For this review, use the dimensioned drawing (mm, ordinates from the lowest corner) and the shaded views. A direction names the side the tool comes from. Coordinates: 2 decimals unless noted, no trailing zeros. Loops run counter-clockwise (first coordinate to the right, second up) from the corner with the lowest first, then second, coordinate; pieces in that order, holes last. Notation, with made-up numbers: M 81,-23 L 125,-23 A27 cw 125,5 Z; hole C 69.5,72.25 d7. An arc over 180 degrees is marked long. Use CSV: the item, a comma, the result in double quotes. Start each with the question number.
1. Clearance check with flat-ended pins moving along their axes: P1, Ø10, axis at x = 8.5, y = 6.5, coming from the +Z side; P2, Ø14, axis at x = 3, y = 55, coming from the +Z side; P3, Ø8, axis at x = 32.5, z = 27.5, coming from the -Y side. State where each tip first meets the part, or that it passes through.
2. Add section A-A, the plane y = 31. Write out the cut boundary in (x, z).
3. Draft analysis for pull direction Y (two halves, no side actions). For the marked faces 4, 5 and 6, state which applies: +Y half, -Y half, draft (parallel to the pull), parting line (faces both ways), or undercut.
4. Tool access review of the marked faces 1, 2 and 3: name each direction out of +Z, -Z, +X, -X, +Y, -Y from which nothing blocks a thin tool from reaching the whole face with its end or side.
5. For L1, parallel to Y at x = 26, z = 4.5; L2, parallel to X at y = 25, z = 8; L3, parallel to Y at x = 17, z = 28, list the stretches that pass through material, from the lowest coordinate up.
6. Add section C-C, the plane x = 19.5. Write out the cut boundary in (y, z) (1 decimal).
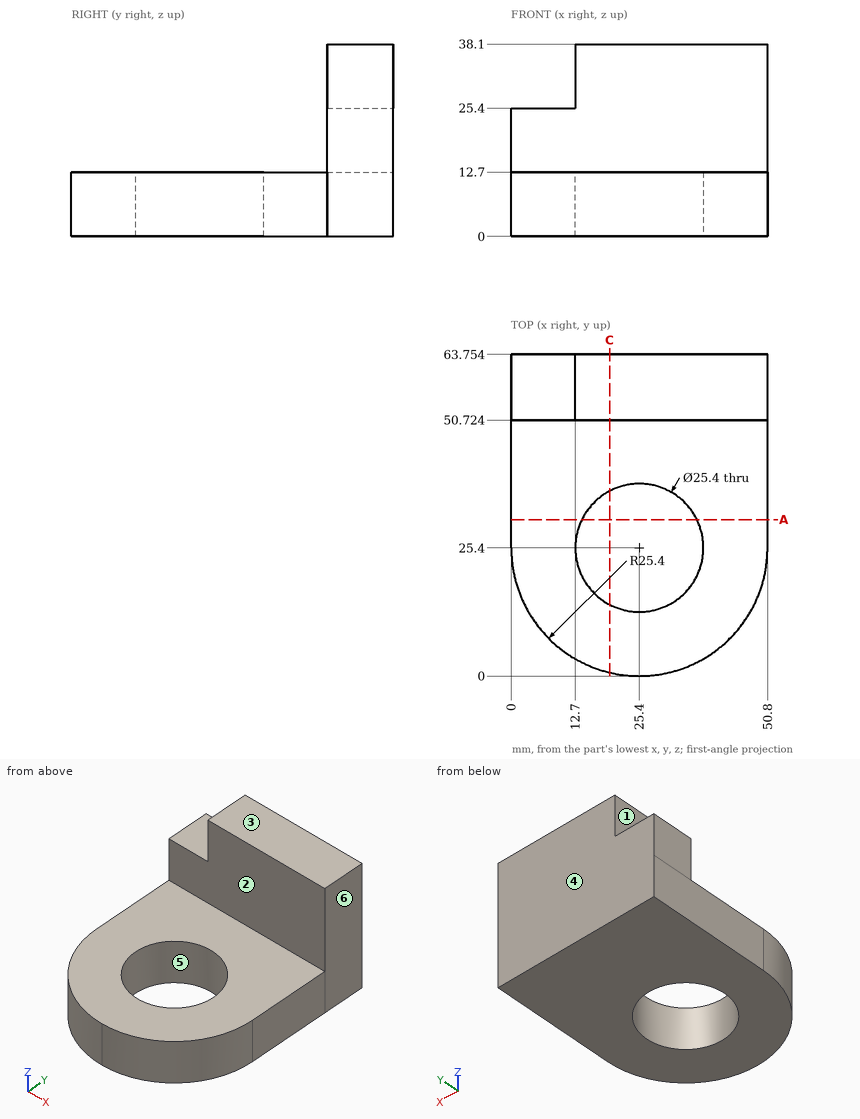
Computed:
1,P1,"stops at z = 12.7"
1,P2,"stops at z = 25.4"
1,P3,"stops at y = 50.72"
2,outline,"M 0,0 L 14,0 L 14,12.7 L 0,12.7 Z; M 36.8,0 L 50.8,0 L 50.8,12.7 L 36.8,12.7 Z"
3,face 4,"+Y half"
3,face 5,"undercut"
3,face 6,"draft"
4,face 1,"+Z, -X, +Y, -Y"
4,face 2,"+Z, +X, -X, -Y"
4,face 3,"+Z, +X, -X, +Y, -Y"
5,L1,"y = 0.01 to 12.71, 38.09 to 63.75"
5,L2,"x = 0 to 12.71, 38.09 to 50.8"
5,L3,"y = 50.72 to 63.75"
6,outline,"M 0.7,0 L 14.2,0 L 14.2,12.7 L 0.7,12.7 Z; M 36.6,0 L 63.8,0 L 63.8,38.1 L 50.7,38.1 L 50.7,12.7 L 36.6,12.7 Z"
